Input: part model. Units: mm. Frame: model coordinates. A direction names the side the tool comes from. Round coordinates to 2 decimals unless told otherwise and drop trailing zeros. Order: outer loops, then holes, each group sorted by start corner. A loop starts at its lowest first (then second) coordinate and runs counter-clockwise, first axis right, second up. Notation, with made-up numbers: M 70,84.5 L 107,84.5 A9 cw 107,96.5 Z; hole C -11.75,-29.75 d1. An arc over 180 degrees is marked long. One line per question, with ' | ' between items.
```python
from build123d import *

# Parameters (mm, degrees)
EXTRUDE_1_DEPTH     = 2
CUT_EXTRUDE_1_DEPTH = 2
FILLET_1_R          = 5
CHAMFER_1_SIZE      = 2


with BuildPart() as part:
    # 草图1 → 凸台-拉伸1 (new body)
    with BuildSketch(Plane(origin=(0, 0, 0), x_dir=(0, 0, -1), z_dir=(1, 0, 0))):
        with BuildLine():
            Line((-20, 2), (-20, 17))
            Line((-20, 17), (20, 17))
            Line((20, 17), (20, 2))
            ThreePointArc((20, 2), (0, 0), (-20, 2))
        make_face()
    extrude(amount=EXTRUDE_1_DEPTH)

    # 草图2 → 切除-拉伸1 (cut)
    with BuildSketch(Plane(origin=(2, 0, 0), x_dir=(0, 0, -1), z_dir=(1, 0, 0))):
        with BuildLine():
            Line((-9.5, 4.832177939), (-9.5, 12.832177939))
            ThreePointArc((-9.5, 12.832177939), (-8, 14.332177939), (-6.5, 12.832177939))
            Line((-6.5, 12.832177939), (-6.5, 4.832177939))
            ThreePointArc((-6.5, 4.832177939), (-8, 3.332177939), (-9.5, 4.832177939))
        make_face()
        with BuildLine():
            Line((9.5, 4.832177939), (9.5, 12.832177939))
            ThreePointArc((9.5, 12.832177939), (8, 14.332177939), (6.5, 12.832177939))
            Line((6.5, 12.832177939), (6.5, 4.832177939))
            ThreePointArc((6.5, 4.832177939), (8, 3.332177939), (9.5, 4.832177939))
        make_face()
    extrude(amount=-CUT_EXTRUDE_1_DEPTH, mode=Mode.SUBTRACT)

    # 圆角1
    fillet_1_edges = [part.edges().sort_by_distance(p)[0] for p in [
        (1, 2, -20),
        (1, 2, 20),
        (1, 17, 20),
        (1, 17, -20),
    ]]
    fillet(fillet_1_edges, radius=FILLET_1_R)

    # 倒角1
    chamfer_1_edges = [part.edges().sort_by_distance(p)[0] for p in [
        (0, 0, 0),
        (0, 2.93152096, -18.801726581),
        (0, 2.93152096, 18.801726581),
        (0, 9.089558112, -20),
        (0, 9.089558112, 20),
        (0, 15.535533906, -18.535533906),
        (0, 15.535533906, 18.535533906),
        (0, 17, 0),
    ]]
    chamfer(chamfer_1_edges, length=CHAMFER_1_SIZE - 0.0001)  # a hair under: the kernel refuses the full size


solid = part.part
```
Item 1: Section query A-A, the plane x = 0.45. Return loops of the section in (y, z).
Report:
outline: M 2.77,-15.54 A3.45 ccw 6.18,-18.45 L 12,-18.45 A3.45 ccw 15.45,-15 L 15.45,15 A3.45 ccw 12,18.45 L 6.18,18.45 A3.45 ccw 2.77,15.54 A99.45 ccw Z; hole M 4.83,-9.5 L 12.83,-9.5 A1.5 ccw 12.83,-6.5 L 4.83,-6.5 A1.5 ccw Z; hole M 4.83,6.5 L 12.83,6.5 A1.5 ccw 12.83,9.5 L 4.83,9.5 A1.5 ccw Z
Item 2: Mould query, pull axis Z, two halves, no side actions, for faces 1 (the flat face through (1, 9, 19)), 2 (the flat face through (1, 9, -9.5)), 3 (the flat face through (1, 16, 0)), 4 (the flat face through (1, 9, -19)). Classes: +Z half, -Z half, draft (parallel to the pull), parting line (faces both ways), or undercut.
Report:
face 1: +Z half | face 2: undercut | face 3: draft | face 4: -Z half
Item 3: Section query B-B, the plane y = 13.75. Give the number of separate pieces and of enclosed holes in the cut face, plus the area to 3 significant figures.
Report:
separate pieces: 3 | enclosed holes: 0 | area: 64.8 mm²
Item 4: Line query: line 1 along Z through (x, y) = (0.4, 8.5); line 2 along Z through (x, y) = (0.6, 12); line 3 along Y through (x, z) = (0.7, -7.5). Output: solid intervals per line, ascending. Write a range as from..to.
Report:
line 1: -18.4..-9.5, -6.5..6.5, 9.5..18.4 | line 2: -18.6..-9.5, -6.5..6.5, 9.5..18.6 | line 3: 1.58..3.42, 14.25..15.7
Item 5: Access query for faces 5 (the flat face through (0, 9, 0)), 6 (the flat face through (1, 9, -6.5)). Directions: +Z, -Z, +X, -X, +Y, -Y. A direction counts if a zero-diameter tool reaches every point of the face in a straight line with its end or side. Return the directions, or none.
Report:
face 5: +Z, -Z, -X, +Y, -Y | face 6: +X, -X
Item 6: First-contact query: pin 1 (4 mm diameter, centred on y = 7.5, z = -2.5, fed in from -X); pin 2 (1 mm diameter, centred on x = 1, y = 9, fed in from +Z). Flat tips, straight axial feed; report the tip coordinate or a pass-through.
Report:
pin 1: x = 0 | pin 2: z = 19.5
